Can you work these out from the model? Positions are in its coordinate system, mm. Face numbers are marked on the shaded views. A direction names the side the tool comes from. Give positions to 0.01 mm unless a question says otherwise; leave off trailing zeros. Loops run counter-clockwise (first coordinate to the right, second up) from the corner with the lowest first, then second, coordinate; pieces in that order, holes last. Notation, with made-up numbers: M 54.25,34.25 L 99.25,34.25 A34 ccw 99.25,73.25 Z; hole C 61.25,78.25 d5. An arc over 180 degrees is marked long. One line per item, written item: value. Start each with the question number.
from build123d import *

# Parameters (mm, degrees)
BOSS_EXTRUDE1_DEPTH   = 15
BOSS_EXTRUDE1_2_DEPTH = 15
BOSS_EXTRUDE2_DEPTH   = 20
SKETCH2_R             = 2.25
CUT_EXTRUDE2_DEPTH    = 12.5


with BuildPart() as part:
    # Sketch1 → Boss-Extrude1 (new, symmetric)
    with BuildSketch(Plane.XY):
        with BuildLine():
            Line((0, 16.97357793), (0, 0))
            Line((0, 0), (28.405213846, 0))
            Line((28.405213846, 0), (21.707328852, 5))
            Line((21.707328852, 5), (40, 5))
            Line((40, 5), (40, 14.47357793))
            Line((40, 14.47357793), (27.5, 14.47357793))
            ThreePointArc((27.5, 14.47357793), (18.661165235, 18.134743165), (15, 26.97357793))
            Line((15, 26.97357793), (10, 26.97357793))
            Line((10, 26.97357793), (10, 16.97357793))
            Line((10, 16.97357793), (0, 16.97357793))
        make_face()
    extrude(amount=BOSS_EXTRUDE1_DEPTH, both=True)



with BuildPart() as body_2:
    # Sketch1 → Boss-Extrude1 2 (new, symmetric)
    with BuildSketch(Plane.XY):
        with BuildLine():
            Line((50, 14.47357793), (50, 5))
            Line((50, 5), (65.219288167, 5))
            Line((65.219288167, 5), (61.486766629, 0))
            Line((61.486766629, 0), (90, 0))
            Line((90, 0), (90, 16.97357793))
            Line((90, 16.97357793), (80, 16.97357793))
            Line((80, 16.97357793), (80, 26.97357793))
            Line((80, 26.97357793), (75, 26.97357793))
            ThreePointArc((75, 26.97357793), (71.338834765, 18.134743165), (62.5, 14.47357793))
            Line((62.5, 14.47357793), (50, 14.47357793))
        make_face()
    extrude(amount=BOSS_EXTRUDE1_2_DEPTH, both=True)


with BuildPart() as part_1:
    add(part.part)

    add(body_2.part)  # Boss-Extrude2 merges body 2
    # Sketch1_3 → Boss-Extrude2 (add, symmetric)
    with BuildSketch(Plane.XY):
        with BuildLine():
            Line((40, 14.47357793), (40, 5))
            Line((40, 5), (50, 5))
            Line((50, 5), (50, 14.47357793))
            Line((50, 14.47357793), (62.5, 14.47357793))
            ThreePointArc((62.5, 14.47357793), (71.338834765, 18.134743165), (75, 26.97357793))
            Line((75, 26.97357793), (70, 26.97357793))
            ThreePointArc((70, 26.97357793), (62.5, 19.47357793), (55, 26.97357793))
            Line((55, 26.97357793), (35, 26.97357793))
            ThreePointArc((35, 26.97357793), (27.5, 19.47357793), (20, 26.97357793))
            Line((20, 26.97357793), (15, 26.97357793))
            ThreePointArc((15, 26.97357793), (18.661165235, 18.134743165), (27.5, 14.47357793))
            Line((27.5, 14.47357793), (40, 14.47357793))
        make_face()
    extrude(amount=BOSS_EXTRUDE2_DEPTH, both=True)

    # Sketch2 → Cut-Extrude2 (cut)
    with BuildSketch(Plane(origin=(0, 26.97357793, 0), x_dir=(1, 0, 0), z_dir=(0, 1, 0))):
        with Locations(Location((14.617344239, 7.5, 0), (0, 0, 180))):
            Circle(SKETCH2_R)
        with Locations(Location((45, 15, 0), (0, 0, 180))):
            Circle(SKETCH2_R)
        with Locations((45, -15)):
            Circle(SKETCH2_R)
        with Locations((14.617344239, -7.5)):
            Circle(SKETCH2_R)
        with Locations(Location((75.511403754, 7.5, 0), (0, 0, 180))):
            Circle(SKETCH2_R)
        with Locations(Location((75.511403754, -7.5, 0), (0, 0, 180))):
            Circle(SKETCH2_R)
    extrude(amount=-CUT_EXTRUDE2_DEPTH, mode=Mode.SUBTRACT)


solid = part_1.part
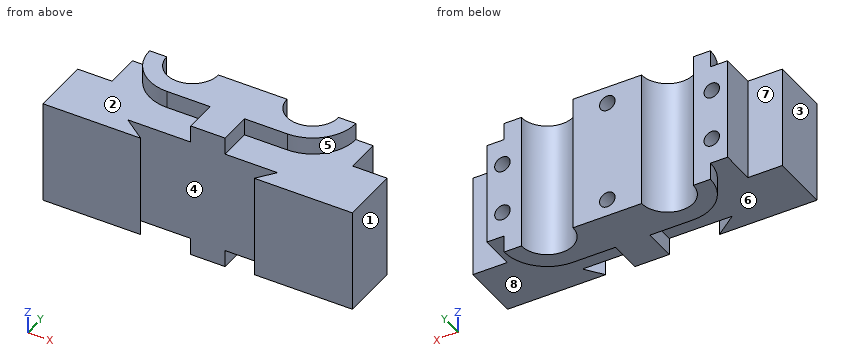
Q1. For P1, Ø4, axis at x = 53.5, z = -16.5, coming from the -Y side; P2, Ø3, axis at x = 17, z = 2.5, coming from the -Y side; P3, Ø2, axis at x = 45.5, z = 15.5, coming from the +Y side; P4, Ø1.5, axis at x = 33, z = -18.5, coming from the -Y side, each with a flat end and sliding along its axis, tell me the tip position at first contact or that it passes through.
Q2. If we mould it in two halves opening along X, with no side actions, what happens to the marked faces 1, 2, 3 and 4? For each: released by +X, released by -X, zero draft, split by the parting line, or undercut.
Q3. If we section it at D-D, the plane x = 57: Write out the boundary of the cut face in (y, z), plus the area to 3 significant figures.
Q4. If we section it at A-A, the plane y = 22.25: Give the number of separate pieces and of enclosed holes in the cut face, plus the area to 3 significant figures.
Q5. Which directions (+Z, -Z, +X, -X, +Y, -Y) give clear straight access to the entire face, cutting with the end or side of a thin tool? Please do the marked faces 5, 6, 7 and 8.
Q6. I need wall thicknesses on line 1 along Z through (x, y) = (45, 23.75); line 2 along Z through (x, y) = (14.5, 17); line 3 along X through (y, z) = (26, 1). Which ranges of each line are inside material? Lowest first, please.
Q7. If we section it at C-C, the plane y = 10.25: Write out the boundary of the cut face in (x, z).
Q8. If we section it at B-B, the plane z = 3: Write out the boundary of the cut face in (x, y), plus the area to 3 significant figures.
Response:
1. P1: y = 5
1. P2: y = 0
1. P3: y = 14.47
1. P4: y = 14.47
2. face 1: released by +X
2. face 2: zero draft
2. face 3: released by -X
2. face 4: undercut
3. outline: M 5,-15 L 14.47,-15 L 14.47,-20 L 21.87,-20 L 21.87,20 L 14.47,20 L 14.47,15 L 5,15 Z
3. area: 580 mm^2
4. separate pieces: 3
4. enclosed holes: 6
4. area: 1,650 mm^2
5. face 5: +Z, +X, -Y
5. face 6: -Z, -X, -Y
5. face 7: +Z, -Z, -X, +Y
5. face 8: -Z, +X, -Y
6. line 1: -20 to -17.25, -12.75 to 12.75, 17.25 to 20
6. line 2: -15 to -9.75, -5.25 to 5.25, 9.75 to 15
6. line 3: 10 to 20.06, 34.94 to 55.06, 69.94 to 80
7. outline: M 0,-15 L 40,-15 L 40,-20 L 50,-20 L 50,-15 L 90,-15 L 90,15 L 50,15 L 50,20 L 40,20 L 40,15 L 0,15 Z
8. outline: M 0,0 L 28.41,0 L 21.71,5 L 65.22,5 L 61.49,0 L 90,0 L 90,16.97 L 80,16.97 L 80,26.97 L 70,26.97 A7.5 cw 55,26.97 L 35,26.97 A7.5 cw 20,26.97 L 10,26.97 L 10,16.97 L 0,16.97 Z
8. area: 1,860 mm^2
